```python
from build123d import *

# Parameters (mm, degrees)
F1_DEPTH  = 16.5
F3_DEPTH  = 2.4
F5_DEPTH  = 2.4
F6_R      = 2.75
F7_DEPTH  = 21.301
F8_SIZE   = 1
F9_R      = 6.5
F10_DEPTH = 4
F11_R     = 6.5
F12_DEPTH = 4


with BuildPart() as f1:
    # F0 (on Front) → F1 (new body)
    with BuildSketch(Plane.XZ):
        with BuildLine():
            Line((10.8, 4.99389), (-10.8, 4.99389))
            Line((-10.8, 4.99389), (-10.8, -14.20611))
            ThreePointArc((-10.8, -14.20611), (0, -25.00611), (10.8, -14.20611))
            Line((10.8, -14.20611), (10.8, 4.99389))
        make_face()
    extrude(amount=F1_DEPTH)

    # F2 (on face) → F3 (join)
    with BuildSketch(Plane.XZ.offset(16.5)):
        with BuildLine():
            Line((10.8, 4.99389), (10.8, -14.20611))
            ThreePointArc((10.8, -14.20611), (0, -25.00611), (-10.8, -14.20611))
            Line((-10.8, -14.20611), (-10.8, 4.99389))
            Line((-10.8, 4.99389), (-16.4, 4.99389))
            Line((-16.4, 4.99389), (-16.4, -13.60611))
            ThreePointArc((-16.4, -13.60611), (0, -30.00611), (16.4, -13.60611))
            Line((16.4, -13.60611), (16.4, 4.99389))
            Line((16.4, 4.99389), (10.8, 4.99389))
        make_face()
        with BuildLine():
            ThreePointArc((-10.8, -14.20611), (0, -25.00611), (10.8, -14.20611))
            Line((10.8, -14.20611), (10.8, 4.99389))
            Line((10.8, 4.99389), (-10.8, 4.99389))
            Line((-10.8, 4.99389), (-10.8, -14.20611))
        make_face()
    extrude(amount=F3_DEPTH)

    # F4 (on face) → F5 (join)
    with BuildSketch(Plane(origin=(0, 0, 0), x_dir=(-1, 0, 0), z_dir=(0, 1, 0))):
        with BuildLine():
            Line((16.4, 4.99389), (-16.4, 4.99389))
            Line((-16.4, 4.99389), (-16.4, -13.60611))
            ThreePointArc((-16.4, -13.60611), (0, -30.00611), (16.4, -13.60611))
            Line((16.4, -13.60611), (16.4, 4.99389))
        make_face()
    extrude(amount=F5_DEPTH)

    # F6 (on face) → F7 (cut, through all)
    with BuildSketch(Plane(origin=(0, 2.4, 0), x_dir=(-1, 0, 0), z_dir=(0, 1, 0))):
        with Locations((0, -13.60611)):
            Circle(F6_R)
    extrude(amount=-F7_DEPTH, mode=Mode.SUBTRACT)

    # F8
    f8_edges = [f1.edges().sort_by_distance(p)[0] for p in [
        (0, -16.5, -30.00611),
        (0, 0, -30.00611),
    ]]
    chamfer(f8_edges, length=F8_SIZE)

    # F9 (on face) → F10 (cut)
    with BuildSketch(Plane(origin=(0, 2.4, 0), x_dir=(-1, 0, 0), z_dir=(0, 1, 0))):
        with Locations((0, -13.60611)):
            Circle(F9_R)
    extrude(amount=-F10_DEPTH, mode=Mode.SUBTRACT)

    # F11 (on face) → F12 (cut)
    with BuildSketch(Plane.XZ.offset(18.9)):
        with Locations((0, -13.60611)):
            Circle(F11_R)
    extrude(amount=-F12_DEPTH, mode=Mode.SUBTRACT)


solid = f1.part
```
Geometry check sheet. Reference: the model listing, model coordinates, mm. A direction names the side the tool comes from. Round coordinates to 2 decimals unless told otherwise and drop trailing zeros. Loops run counter-clockwise (first coordinate to the right, second up) from the corner with the lowest first, then second, coordinate; pieces in that order, holes last. Notation, with made-up numbers: (-8.75, 8) - (14.25, 8) arc R28 cw to (14.25, 39) - close; hole circle Ø10 at (-33, 80). An arc over 180 degrees is marked (long way). Use a Markdown table: item, result.
Q1. Material ranges on line 1 (Z direction, x = 0, y = 1.4); line 2 (Z direction, x = 0, y = -11.25); line 3 (X direction, y = -13.5, z = 1.5), recorded low to high.
Solutions:
| item | result |
|---|---|
| line 1 | z = -30.01 to -20.11, -7.11 to 4.99 |
| line 2 | z = -25.01 to -16.36, -10.86 to 4.99 |
| line 3 | x = -10.8 to 10.8 |
Q2. Go/stop test with flat-tipped pins: P1, Ø5, axis at x = -10, y = -11, coming from the -Z side; P2, Ø10, axis at y = -4, z = -22.5, coming from the -X side; P3, Ø8, axis at x = -6.5, y = -10.5, coming from the -Z side. Record where each tip stops, or that it passes through.
Solutions:
| item | result |
|---|---|
| P1 | stops at z = -21.98 |
| P2 | stops at x = -14.42 |
| P3 | stops at z = -24.71 |
Q3. Access from +Z, -Z, +X, -X, +Y, -Y to the whole of each face (thin tool, end or side, straight path). Record for faces 1 (the cylindrical face through (-0.237, -8.134, -25.003)), 2 (the cylindrical face through (2.999, -16.928, -19.373)), 3 (the flat face through (-15.9, -17, -4.2)), 4 (the cylindrical face through (-2.999, 0.428, -19.373)), 5 (the flat face through (10.8, -8, -5)).
Solutions:
| item | result |
|---|---|
| face 1 | -Z |
| face 2 | -Y |
| face 3 | +Z, -Z, -X |
| face 4 | +Y |
| face 5 | +Z, -Z, +X |
Q4. Cross-section at A-A on y = -11.5. Record the cut outline in (x, z), plus the area to 3 significant figures.
Solutions:
| item | result |
|---|---|
| outline | (-10.8, -14.21) arc R10.8 ccw to (10.8, -14.21) - (10.8, 4.99) - (-10.8, 4.99) - close; hole circle Ø5.5 at (0, -13.61) |
| area | 574 mm2 |
Q5. Cross-section at B-B on x = 0. Record the cut outline in (y, z).
Solutions:
| item | result |
|---|---|
| outline | (-18.9, -30.01) - (-17.5, -30.01) - (-16.5, -29.01) - (-16.5, -25.01) - (0, -25.01) - (0, -29.01) - (1, -30.01) - (2.4, -30.01) - (2.4, -20.11) - (-1.6, -20.11) - (-1.6, -16.36) - (-14.9, -16.36) - (-14.9, -20.11) - (-18.9, -20.11) - close; (-18.9, -7.11) - (-14.9, -7.11) - (-14.9, -10.86) - (-1.6, -10.86) - (-1.6, -7.11) - (2.4, -7.11) - (2.4, 4.99) - (-18.9, 4.99) - close |
Q6. Cross-section at C-C on z = -6.5. Record the cut outline in (x, y).
Solutions:
| item | result |
|---|---|
| outline | (-16.4, -18.9) - (16.4, -18.9) - (16.4, -17.5) - (15.4, -16.5) - (10.8, -16.5) - (10.8, 0) - (15.4, 0) - (16.4, 1) - (16.4, 2.4) - (-16.4, 2.4) - (-16.4, 1) - (-15.4, 0) - (-10.8, 0) - (-10.8, -16.5) - (-15.4, -16.5) - (-16.4, -17.5) - close |
Q7. Draft check along Y on faces 6 (the flat face through (15.9, 0.5, -4.2)), 7 (the flat face through (-4, -18.9, -8)), 8 (the flat face through (16.4, 2, -4)), 9 (the flat face through (4, 2.4, -8)). Enter one of: released by +Y, released by -Y, zero draft, split by the parting line, or undercut.
Solutions:
| item | result |
|---|---|
| face 6 | undercut |
| face 7 | released by -Y |
| face 8 | zero draft |
| face 9 | released by +Y |
